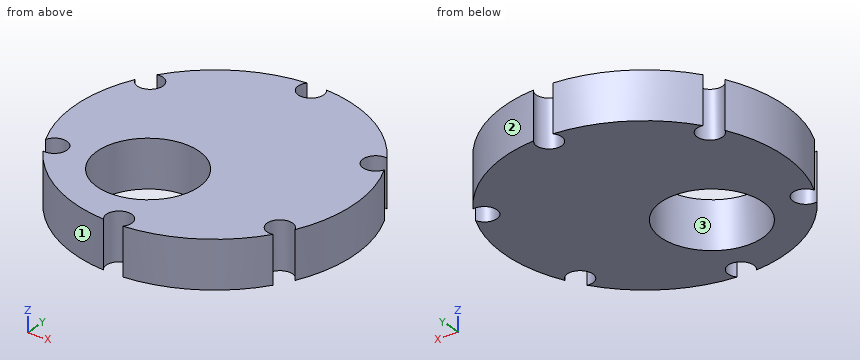
```python
from build123d import *

# Parameters (mm, degrees)
SKETCH1_R           = 16.5
BOSS_EXTRUDE1_DEPTH = 5.6
SKETCH2_R           = 1.5
CUT_EXTRUDE1_DEPTH  = 24.997083156
SKETCH3_R           = 6
CUT_EXTRUDE2_DEPTH  = 24.969375894


with BuildPart() as part:
    # Sketch1 → Boss-Extrude1 (new body)
    with BuildSketch(Plane.XY):
        Circle(SKETCH1_R)
    extrude(amount=BOSS_EXTRUDE1_DEPTH)

    # Sketch2 → Cut-Extrude1 (cut, through all)
    with BuildSketch(Plane.XY.offset(5.6)):
        with Locations((0, 15.5)):
            Circle(SKETCH2_R)
        with Locations((13.423393759, 7.75)):
            Circle(SKETCH2_R)
        with Locations((13.423393759, -7.75)):
            Circle(SKETCH2_R)
        with Locations((0, -15.5)):
            Circle(SKETCH2_R)
        with Locations((-13.423393759, -7.75)):
            Circle(SKETCH2_R)
        with Locations((-13.423393759, 7.75)):
            Circle(SKETCH2_R)
    extrude(amount=-CUT_EXTRUDE1_DEPTH, mode=Mode.SUBTRACT)

    # Sketch3 → Cut-Extrude2 (cut, through all)
    with BuildSketch(Plane.XY.offset(5.6)):
        with Locations((-3.5, -6.062177826)):
            Circle(SKETCH3_R)
    extrude(amount=-CUT_EXTRUDE2_DEPTH, mode=Mode.SUBTRACT)


solid = part.part
```
Geometry: final body of the model. Coordinates: model frame, mm. Face numbers are marked on the shaded views. Coordinates: 2 decimals unless noted, no trailing zeros. Order: outer loops, then holes, each group sorted by start corner. A loop starts at its lowest first (then second) coordinate and runs counter-clockwise, first axis right, second up. Notation, with made-up numbers: (79, 21.5) - (126, 21.5) arc R12 cw to (126, 44.5) - close; hole circle Ø3 at (22, -24). An arc over 180 degrees is marked (long way). Write each question's results on one line, items separated by ' | '.
1) Section A-A, the plane x = -7.5. Return loops of the section in (y, z), plus the area to 3 significant figures.
Results list:
outline: (-14.7, 0) - (-10.53, 0) - (-10.53, 5.6) - (-14.7, 5.6) - close; (-1.59, 0) - (14.7, 0) - (14.7, 5.6) - (-1.59, 5.6) - close | area: 115 mm^2
2) Pull-direction query (X, two-part tool) for the marked faces 1, 2 and 3; classes: pulls with the +X half, pulls with the -X half, needs draft (parallel to the pull), parting line crosses it, or undercut.
Results list:
face 1: pulls with the -X half | face 2: pulls with the +X half | face 3: undercut
3) Line query: line 1 (X direction, y = -7, z = 4.8); line 2 (X direction, y = -10.5, z = 1.65); line 3 (Y direction, x = -2.5, z = 3.95). Output: solid intervals per line, ascending. Write a range as from..to.
Results list:
line 1: -14.94..-14.72, -12.12..-9.43, 2.43..12.12, 14.72..14.94 | line 2: -12.73..-7.54, 0.54..12.73 | line 3: -16.31..-11.98, -0.15..16.31
4) Section D-D, the plane y = 7.75. Return loops of the section in (x, z), plus the area to 3 significant figures.
Results list:
outline: (-11.92, 0) - (11.92, 0) - (11.92, 5.6) - (-11.92, 5.6) - close | area: 134 mm^2
5) Section B-B, the plane y = -7.75. Return loops of the section in (x, z), plus the area to 3 significant figures.
Results list:
outline: (-11.92, 0) - (-9.26, 0) - (-9.26, 5.6) - (-11.92, 5.6) - close; (2.26, 0) - (11.92, 0) - (11.92, 5.6) - (2.26, 5.6) - close | area: 69.1 mm^2
6) Section C-C, the plane z = 1.3. Return loops of the section in (x, y), plus the area to 3 significant figures.
Results list:
outline: (-14.83, -7.23) arc R1.5 cw (long way) to (-13.68, -9.23) arc R16.5 ccw to (-1.15, -16.46) arc R1.5 cw (long way) to (1.15, -16.46) arc R16.5 ccw to (13.68, -9.23) arc R1.5 cw (long way) to (14.83, -7.23) arc R16.5 ccw to (14.83, 7.23) arc R1.5 cw (long way) to (13.68, 9.23) arc R16.5 ccw to (1.15, 16.46) arc R1.5 cw (long way) to (-1.15, 16.46) arc R16.5 ccw to (-13.68, 9.23) arc R1.5 cw (long way) to (-14.83, 7.23) arc R16.5 ccw to start; hole circle Ø12 at (-3.5, -6.06) | area: 705 mm^2
7) Pin query (flat end, axial travel): pin 1 (1 mm diameter, centred on y = 12.5, z = 1, fed in from +X); pin 2 (1 mm diameter, centred on x = 0.5, z = 2, fed in from +Y). Return the tip coordinate at first contact, or that it passes through.
Results list:
pin 1: x = 11.32 | pin 2: y = 14.38
